The model under review builds one solid part; all positions refer to its coordinate system, in mm. Give positions to 0.01 mm unless a question says otherwise; leave off trailing zeros. Write each loop counter-clockwise with the first axis right and the second up, starting at its lowest first coordinate (ties: lowest second). Pieces come first, ordered by that corner, then holes. Notation, with made-up numbers: (27.25, 10.5) - (78.25, 10.5) arc R32 cw to (78.25, 45.5) - close; hole circle Ø4 at (41, -26.5). An arc over 180 degrees is marked (long way). Write item = value, one per line.
```python
from build123d import *

# Parameters (mm, degrees)
SKETCH_1_R      = 1.75
EXTRUDE_1_DEPTH = 3


with BuildPart() as part:
    # 草圖1 → 伸長1 (new body)
    with BuildSketch(Plane.XY):
        with BuildLine():
            Line((-6.666666667, 7.5), (20, 7.5))
            ThreePointArc((20, 7.5), (27.5, 0), (20, -7.5))
            Line((20, -7.5), (-20, -7.5))
            Line((-20, -7.5), (-6.666666667, 7.5))
        make_face()
        with Locations((20, 0)):
            Circle(SKETCH_1_R, mode=Mode.SUBTRACT)
        with Locations((-6.666666667, 0)):
            Circle(SKETCH_1_R, mode=Mode.SUBTRACT)
        with Locations((6.666666667, 0)):
            Circle(SKETCH_1_R, mode=Mode.SUBTRACT)
    extrude(amount=EXTRUDE_1_DEPTH)


solid = part.part
```
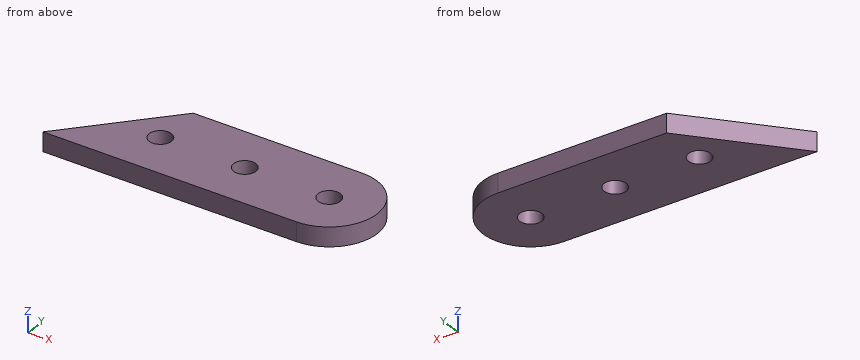
1. For line 1 (X direction, y = -1.25, z = 0.7); line 2 (X direction, y = 1.5, z = 1.3); line 3 (Y direction, x = 6, z = 2.05), list the stretches that pass through material, from the lowest coordinate up. Write a range as from..to.
Findings below:
line_1 = -14.44..-7.89, -5.44..5.44, 7.89..18.78, 21.22..27.4
line_2 = -12..-7.57, -5.77..5.77, 7.57..19.1, 20.9..27.35
line_3 = -7.5..-1.62, 1.62..7.5
2. Take a section at C-C on x = 6. Give the boundary of the cut face in (y, z), and give its area (3 significant figures).
Findings below:
outline = (-7.5, 0) - (-1.62, 0) - (-1.62, 3) - (-7.5, 3) - close; (1.62, 0) - (7.5, 0) - (7.5, 3) - (1.62, 3) - close
area = 35.3 mm²
3. Insertion check: P1, Ø2, axis at x = -7, y = -0.5, coming from the +Z side; P2, Ø1.5, axis at y = 0, z = 0.5, coming from the -X side. Each pin has a flat end and moves straight along its axis. Give the tip position at first contact, or say it passes through.
Findings below:
P1 = through
P2 = -14
4. Take a section at D-D on y = -3.5. Give the boundary of the cut face in (x, z), and give its area (3 significant figures).
Findings below:
outline = (-16.44, 0) - (26.63, 0) - (26.63, 3) - (-16.44, 3) - close
area = 129 mm²
5. Take a section at B-B on y = -1. Give the boundary of the cut face in (x, z), and give its area (3 significant figures).
Findings below:
outline = (-14.22, 0) - (-8.1, 0) - (-8.1, 3) - (-14.22, 3) - close; (-5.23, 0) - (5.23, 0) - (5.23, 3) - (-5.23, 3) - close; (8.1, 0) - (18.56, 0) - (18.56, 3) - (8.1, 3) - close; (21.44, 0) - (27.43, 0) - (27.43, 3) - (21.44, 3) - close
area = 99.1 mm²
6. Take a section at A-A on z = 1.95. Give the boundary of the cut face in (x, y), and give its area (3 significant figures).
Findings below:
outline = (-20, -7.5) - (20, -7.5) arc R7.5 ccw to (20, 7.5) - (-6.67, 7.5) - close; hole circle Ø3.5 at (-6.67, 0); hole circle Ø3.5 at (6.67, 0); hole circle Ø3.5 at (20, 0)
area = 559 mm²
